Autodesk Inventor part; units mm, degrees
ref_plane "YZ Plane" through (0, 0, 0) normal (1, 0, 0) x (0, 1, 0)
ref_plane "XZ Plane" through (0, 0, 0) normal (0, 1, 0) x (-1, 0, 0)
ref_plane "XY Plane" through (0, 0, 0) normal (0, 0, 1) x (1, 0, 0)
sketch "Sketch1" plane through (0, 0, 0) normal (0, 0, 1) x (1, 0, 0)
  line L0 (101.6, 0) -> (101.6, -12.7)
  line L1 (101.6, -12.7) -> (0, -12.7)
  line L2 (50.8, 0) -> (0, 0)
  line L3 (50.8, 0) -> (101.6, 0)
  line L4 (0, -12.7) -> (50.8, -12.7)
  line L5 (50.8, -12.7) -> (101.6, -12.7)
  circle A0 centre (25.4, -6.35) radius 1.85
  circle A1 centre (50.8, -6.35) radius 1.85
  circle A2 centre (76.2, -6.35) radius 1.85
  line L6 (0, -12.7) -> (-60, -12.7)
  line L7 (-60, -12.7) -> (-60, 0)
  line L8 (-9.5, 0) -> (-9.5, 13.9)
  line L9 (-9.5, 13.9) -> (0, 13.9)
  line L10 (0, 13.9) -> (0, 0)
  line L11 (-50.5004, 13.8938) -> (-60, 13.8938)
  line L12 (-60, 13.8938) -> (-60, 0)
  line L13 (-50.5004, 13.8938) -> (-53.7504, 13.8938)
  circle A3 centre (-53.7504, 8.8938) radius 1.8542
  line L14 (-9.5, 13.9) -> (-6.2488, 13.9)
  line L15 (-9.5, 8.8962) -> (-9.5, 13.9)
  circle A4 centre (-6.2488, 8.8962) radius 1.8542
  line L16 (-53.7504, 13.8938) -> (-50.5004, 13.8938)
  circle A5 centre (-53.7504, -1.1062) radius 1.8542
  circle A6 centre (-6.2488, -1.1) radius 1.8542
  line L17 (-9.5, 0) -> (-50.5004, 0)
  line L18 (-50.5004, 13.8938) -> (-50.5004, 0)
  line L19 (0, 0) -> (0, -12.7)
  line L20 (0, 0) -> (101.6, 0)
  line L21 (101.6, 0) -> (101.6, -12.7)
  line L22 (101.6, -12.7) -> (0, -12.7)
  line L23 (-60, 13.8938) -> (-60, -12.7)
  line L24 (-60, -12.7) -> (0, -12.7)
  line L25 (0, -12.7) -> (0, 13.9)
  line L26 (0, 13.9) -> (-9.5, 13.9)
  line L27 (-9.5, 0) -> (-50.5004, 0)
  line L28 (-50.5004, 13.8938) -> (-60, 13.8938)
  dimension "d0" = 101.6
  dimension "d1" = 12.7
  dimension "d2" = 3.7
  dimension "d3" = 3.7
  dimension "d4" = 3.7
  dimension "d5" = 60
  dimension "d6" = 9.5
  dimension "d7" = 13.9
  dimension "d8" = 9.4996
  dimension "d9" = 13.8938
  dimension "d12" = 3.7084
  dimension "d15" = 3.7084
  dimension "d17" = 3.7084
  dimension "d19" = 3.7084
extrude "Extrusion1" add sketch "Sketch1" along normal blind 6.35
properties part number "flapperservomount"
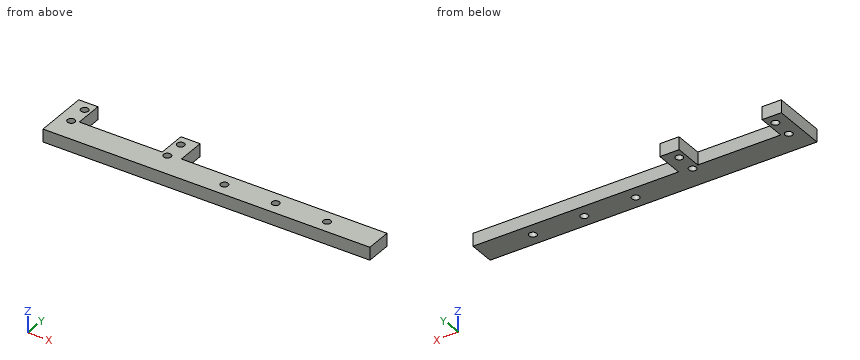
The listing builds one solid part. Answer for the finished solid, in the listing's coordinates (mm). Round coordinates to 2 decimals unless told otherwise and drop trailing zeros. Order: outer loops, then holes, each group sorted by start corner. A loop starts at its lowest first (then second) coordinate and runs counter-clockwise, first axis right, second up. Notation, with made-up numbers: (7, -10) -> (18, -10) arc R17 ccw to (18, 20) -> close; hole circle Ø1 at (61.5, 0). An arc over 180 degrees is marked (long way). Answer as CSV lines item,"result".
Q1. Consider line 1 (X direction, y = 9, z = 4.75); line 2 (Y direction, x = 50.8, z = 1.75); line 3 (X direction, y = -1.75, z = 6). Determine where each line is inside the solid, lowest interval first. Write a range as from..to.
Computed values:
line 1,"x = -60..-55.6, -51.9..-50.5, -9.5..-8.1, -4.4..0"
line 2,"y = -12.7..-8.2, -4.5..0"
line 3,"x = -60..-55.49, -52.01..-7.99, -4.51..101.6"
Q2. A cutting plane is placed at D-D on x = -24. Determine the outline of the cut face in (y, z).
Computed values:
outline,"(-12.7, 0) -> (0, 0) -> (0, 6.35) -> (-12.7, 6.35) -> close"
Q3. Given pin 1 (1.5 mm diameter, centred on x = 10, z = 2, fed in from +Y); pin 2 (3 mm diameter, centred on y = 7, z = 1.5, fed in from +X); pin 3 (5 mm diameter, centred on x = -53.75, y = -1.11, fed in from -Z), each flat-ended and moving along its own axis, determine where each tip first touches the part or whether it passes through.
Computed values:
pin 1,"stops at y = 0"
pin 2,"stops at x = 0"
pin 3,"stops at z = 0"
Q4. A cutting plane is placed at B-B on x = 76.2. Determine the outline of the cut face in (y, z), plus the area to 4 significant figures.
Computed values:
outline,"(-12.7, 0) -> (-8.2, 0) -> (-8.2, 6.35) -> (-12.7, 6.35) -> close; (-4.5, 0) -> (0, 0) -> (0, 6.35) -> (-4.5, 6.35) -> close"
area,"57.15 mm^2"
Q5. A cutting plane is placed at C-C on z = 4.5. Determine the outline of the cut face in (x, y).
Computed values:
outline,"(-60, -12.7) -> (101.6, -12.7) -> (101.6, 0) -> (0, 0) -> (0, 13.9) -> (-9.5, 13.9) -> (-9.5, 0) -> (-50.5, 0) -> (-50.5, 13.89) -> (-60, 13.89) -> close; hole circle Ø3.71 at (-53.75, -1.11); hole circle Ø3.71 at (-53.75, 8.89); hole circle Ø3.71 at (-6.25, -1.1); hole circle Ø3.71 at (-6.25, 8.9); hole circle Ø3.7 at (25.4, -6.35); hole circle Ø3.7 at (50.8, -6.35); hole circle Ø3.7 at (76.2, -6.35)"
Q6. A cutting plane is placed at A-A on y = -6.35. Determine the outline of the cut face in (x, z).
Computed values:
outline,"(-60, 0) -> (23.55, 0) -> (23.55, 6.35) -> (-60, 6.35) -> close; (27.25, 0) -> (48.95, 0) -> (48.95, 6.35) -> (27.25, 6.35) -> close; (52.65, 0) -> (74.35, 0) -> (74.35, 6.35) -> (52.65, 6.35) -> close; (78.05, 0) -> (101.6, 0) -> (101.6, 6.35) -> (78.05, 6.35) -> close"
